```python
from build123d import *

# Parameters (mm, degrees)
BOSS_EXTRUDE1_DEPTH = 1.5
SKETCH2_R           = 4
BOSS_EXTRUDE2_DEPTH = 5.5
FILLET1_R           = 2.54


with BuildPart() as part:
    # Sketch1 → Boss-Extrude1 (new body)
    with BuildSketch(Plane.XY):
        with BuildLine():
            Line((-3.81, 10), (3.81, 10))
            ThreePointArc((3.81, 10), (3.6, 6.235382907), (6.755254038, 8.299556788))
            Line((6.755254038, 8.299556788), (10.565254038, 1.700443212))
            ThreePointArc((10.565254038, 1.700443212), (7.2, 0), (10.565254038, -1.700443212))
            Line((10.565254038, -1.700443212), (6.755254038, -8.299556788))
            ThreePointArc((6.755254038, -8.299556788), (3.6, -6.235382907), (3.81, -10))
            Line((3.81, -10), (-3.81, -10))
            ThreePointArc((-3.81, -10), (-3.6, -6.235382907), (-6.755254038, -8.299556788))
            Line((-6.755254038, -8.299556788), (-10.565254038, -1.700443212))
            ThreePointArc((-10.565254038, -1.700443212), (-7.2, 0), (-10.565254038, 1.700443212))
            Line((-10.565254038, 1.700443212), (-6.755254038, 8.299556788))
            ThreePointArc((-6.755254038, 8.299556788), (-3.6, 6.235382907), (-3.81, 10))
        make_face()
    extrude(amount=BOSS_EXTRUDE1_DEPTH)

    # Sketch2 → Boss-Extrude2 (add)
    with BuildSketch(Plane.XY.offset(1.5)):
        Circle(SKETCH2_R)
    extrude(amount=BOSS_EXTRUDE2_DEPTH)

    # Fillet1
    fillet1_edges = [part.edges().sort_by_distance(p)[0] for p in [
        (-4, 0, 7),
    ]]
    fillet(fillet1_edges, radius=FILLET1_R)


solid = part.part
```
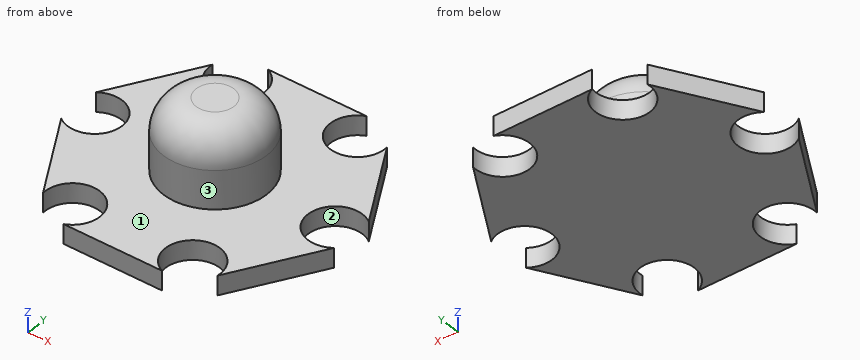
Geometry check sheet. Reference: the model listing, model coordinates, mm. Face numbers are marked on the shaded views. Give positions to 0.01 mm unless a question says otherwise; leave off trailing zeros. Write each loop counter-clockwise with the first axis right and the second up, starting at its lowest first coordinate (ties: lowest second). Pieces come first, ordered by that corner, then holes.
1) Gauge pin test, flat ends, axial feed: pin 1 (3 mm diameter, centred on x = -3.5, z = 5.5, fed in from +Y); pin 2 (4 mm diameter, centred on x = 4.66, y = 8.06, fed in from +Z); pin 3 (4 mm diameter, centred on x = 0.5, y = 4.5, fed in from +Z); pin 4 (5.5 mm diameter, centred on x = -9.31, y = 0, fed in from +Z). Record the tip position at first contact, or that the pin passes through.
2) Material ranges on L1, parallel to Y at x = 3.5, z = 0.5; L2, parallel to Z at x = 7, y = 6; L3, parallel to Y at x = 7.75, z = 1, recorded low to high.
3) Release check for a two-part mould opening along Y. For the marked faces 1, 2 and 3 record: pulls with the +Y half, pulls with the -Y half, needs draft (parallel to the pull), parting line crosses it, or undercut.
4) Section check C-C, the plane z = 3.5. Record the boundary of the cut face in (x, y), and give its area (3 significant figures).
5) Section check A-A, the plane x = -8. Record the boundary of the cut face in (y, z).
6) Section check D-D, the plane x = -3. State how many separate pieces and enclosed holes the cut face has, and give its area (3 significant figures).
7) Section check B-B, the plane y = -7.5. Record the boundary of the cut face in (x, z).
Computed:
1. pin 1: stops at y = 3.35
1. pin 2: passes through
1. pin 3: stops at z = 6.76
1. pin 4: stops at z = 1.5
2. L1: y = -10 to -9.83, -6.3 to 6.3, 9.83 to 10
2. L2: z = 0 to 1.5
2. L3: y = -6.58 to -1.42, 1.42 to 6.58
3. face 1: needs draft
3. face 2: undercut
3. face 3: parting line crosses it
4. outline: circle Ø8 at (0, 0)
4. area: 50.3 mm2
5. outline: (-6.14, 0) - (-1.66, 0) - (-1.66, 1.5) - (-6.14, 1.5) - close; (1.66, 0) - (6.14, 0) - (6.14, 1.5) - (1.66, 1.5) - close
6. separate pieces: 3
6. enclosed holes: 0
6. area: 46.3 mm2
7. outline: (-7.22, 0) - (-6.69, 0) - (-6.69, 1.5) - (-7.22, 1.5) - close; (-2.62, 0) - (2.62, 0) - (2.62, 1.5) - (-2.62, 1.5) - close; (6.69, 0) - (7.22, 0) - (7.22, 1.5) - (6.69, 1.5) - close
